Model file for the job. Use its own axes, mm. A direction names the side the tool comes from. Coordinates: 2 decimals unless noted, no trailing zeros. Loops run counter-clockwise (first coordinate to the right, second up) from the corner with the lowest first, then second, coordinate; pieces in that order, holes last.
from build123d import *

# Parameters (mm, degrees)
ESBO_O1_R                  = 2.5
ESBO_O1_R_2                = 4
RESSALTO_EXTRUS_O1_DEPTH   = 4
ESBO_O2_R                  = 13.5
ESBO_O2_R_2                = 10.5
RESSALTO_EXTRUS_O2_DEPTH   = 5
ESBO_O3_R                  = 7
ESBO_O3_R_2                = 4
RESSALTO_EXTRUS_O3_DEPTH   = 9
ESBO_O4_R                  = 1.5
CORTE_EXTRUS_O1_DEPTH      = 14.5
CORTE_EXTRUS_O1_DEPTH_BACK = 14.5
ESBO_O5_R                  = 1.5
CORTE_EXTRUS_O2_DEPTH      = 24.75
CORTE_EXTRUS_O2_DEPTH_BACK = 24.75


with BuildPart() as part:
    # Esboço1 → Ressalto-extrusão1 (new body)
    with BuildSketch(Plane.XY):
        with BuildLine():
            Line((-18.25, 5.5), (-6.677721963, 11.73277586))
            ThreePointArc((-6.677721963, 11.73277586), (0, 13.5), (6.677721963, 11.73277586))
            Line((6.677721963, 11.73277586), (18.25, 5.5))
            ThreePointArc((18.25, 5.5), (23.75, 0), (18.25, -5.5))
            Line((18.25, -5.5), (6.677721963, -11.73277586))
            ThreePointArc((6.677721963, -11.73277586), (0, -13.5), (-6.677721963, -11.73277586))
            Line((-6.677721963, -11.73277586), (-18.25, -5.5))
            ThreePointArc((-18.25, -5.5), (-23.75, 0), (-18.25, 5.5))
        make_face()
        with Locations((-18.25, 0)):
            Circle(ESBO_O1_R, mode=Mode.SUBTRACT)
        with Locations((18.25, 0)):
            Circle(ESBO_O1_R, mode=Mode.SUBTRACT)
        Circle(ESBO_O1_R_2, mode=Mode.SUBTRACT)
    extrude(amount=RESSALTO_EXTRUS_O1_DEPTH)

    # Esboço2 → Ressalto-extrusão2 (add)
    with BuildSketch(Plane.XY.offset(4)):
        Circle(ESBO_O2_R)
        Circle(ESBO_O2_R_2, mode=Mode.SUBTRACT)
    extrude(amount=RESSALTO_EXTRUS_O2_DEPTH)

    # Esboço3 → Ressalto-extrusão3 (add)
    with BuildSketch(Plane.XY.offset(4)):
        Circle(ESBO_O3_R)
        Circle(ESBO_O3_R_2, mode=Mode.SUBTRACT)
    extrude(amount=RESSALTO_EXTRUS_O3_DEPTH)

    # Esboço4 → Corte-extrusão1 (cut, two sides)
    with BuildSketch(Plane(origin=(0, 0, 0), x_dir=(1, 0, 0), z_dir=(0, 1, 0))) as corte_extrus_o1_sk:
        with Locations((0, -11)):
            Circle(ESBO_O4_R)
    extrude(amount=CORTE_EXTRUS_O1_DEPTH, mode=Mode.SUBTRACT)
    extrude(corte_extrus_o1_sk.sketch, amount=-CORTE_EXTRUS_O1_DEPTH_BACK, mode=Mode.SUBTRACT)

    # Esboço5 → Corte-extrusão2 (cut, two sides)
    with BuildSketch(Plane(origin=(0, 0, 0), x_dir=(0, 0, -1), z_dir=(1, 0, 0))) as corte_extrus_o2_sk:
        with Locations((-11, 0)):
            Circle(ESBO_O5_R)
    extrude(amount=CORTE_EXTRUS_O2_DEPTH, mode=Mode.SUBTRACT)
    extrude(corte_extrus_o2_sk.sketch, amount=-CORTE_EXTRUS_O2_DEPTH_BACK, mode=Mode.SUBTRACT)


solid = part.part
Q1. Slice it at A-A (x = 0). List the corners of the cut face in (y, z).
Answers:
outline: (-13.5, 0) - (-4, 0) - (-4, 9.5) - (-7, 9.5) - (-7, 4) - (-10.5, 4) - (-10.5, 9) - (-13.5, 9) - close; (-7, 12.5) - (-4, 12.5) - (-4, 13) - (-7, 13) - close; (4, 0) - (13.5, 0) - (13.5, 9) - (10.5, 9) - (10.5, 4) - (7, 4) - (7, 9.5) - (4, 9.5) - close; (4, 12.5) - (7, 12.5) - (7, 13) - (4, 13) - close
Q2. Flat gauge pins, fed straight in: P1, Ø6, axis at x = -18.25, y = 0, coming from the +Z side; P2, Ø6, axis at y = 7.5, z = 3, coming from the -X side; P3, Ø8, axis at x = -1, y = -2, coming from the +Z side; P4, Ø1, axis at y = 10.5, z = 2, coming from the +X side. Where does each tip first touch, or does it go through?
Answers:
P1: stops at z = 4
P2: stops at x = -21.41
P3: stops at z = 13
P4: stops at x = 9.89
Q3. Slice it at D-D (y = 0). Count the separate pieces of the cut face and the enclosed holes in it, and give its area (3 significant figures).
Answers:
separate pieces: 6
enclosed holes: 0
area: 184 mm2
Q4. Mould opens along X. For faces 1 (the cylindrical face through (-5.331, -0.575, 9.614)), 2 (the cylindrical face through (6.466, -2.681, 8.437)), 3 (the flat face through (-12.38, -8.66, 1.97)) say: +X half, -X half, draft (parallel to the pull), parting line (faces both ways), or undercut.
Answers:
face 1: draft
face 2: undercut
face 3: -X half
Q5. Slice it at C-C (z = 6.75). List the corners of the cut face in (x, y).
Answers:
outline: circle Ø27 at (0, 0); circle Ø14 at (0, 0); hole circle Ø21 at (0, 0); hole circle Ø8 at (0, 0)
Q6. Slice it at B-B (z = 3.5). List the corners of the cut face in (x, y), and give its area (3 significant figures).
Answers:
outline: (-18.25, -5.5) - (-6.68, -11.73) arc R13.5 ccw to (6.68, -11.73) - (18.25, -5.5) arc R5.5 ccw to (18.25, 5.5) - (6.68, 11.73) arc R13.5 ccw to (-6.68, 11.73) - (-18.25, 5.5) arc R5.5 ccw to start; hole circle Ø5 at (-18.25, 0); hole circle Ø8 at (0, 0); hole circle Ø5 at (18.25, 0)
area: 750 mm2
Q7. Which spindle directions (+Z, -Z, +X, -X, +Y, -Y) get a long thin tool onto all of the face, cutting with end or side? Do faces 4 (the cylindrical face through (-1.5, -5.33, 10.93)), 5 (the flat face through (0, -11, 9)). Say none if no direction does.
Answers:
face 4: +Y, -Y
face 5: +Z
Q8. Drill centre lines: line 1 (Y direction, x = 0, z = 7.25); line 2 (Y direction, x = -1.5, z = 7.75); line 3 (X direction, y = -0.25, z = 2.75). Where is each one in solid material? Low to high.
Answers:
line 1: y = -13.5 to -10.5, -7 to -4, 4 to 7, 10.5 to 13.5
line 2: y = -13.42 to -10.39, -6.84 to -3.71, 3.71 to 6.84, 10.39 to 13.42
line 3: x = -23.74 to -20.74, -15.76 to -3.99, 3.99 to 15.76, 20.74 to 23.74
